from build123d import *

# Parameters (mm, degrees)
F1_DEPTH = 150
F2_R     = 30


with BuildPart() as f1:
    # F0 (on Front) → F1 (new body)
    with BuildSketch(Plane.XZ):
        Polygon((0, 206.360267), (0, 150), (150, 150), (500, 550), (350, 550), (300.684766, 550), align=None)
    extrude(amount=F1_DEPTH)

    # F2
    f2_edges = [f1.edges().sort_by_distance(p)[0] for p in [
        (150.342383, -150, 378.180134),
        (325, -150, 350),
        (325, 0, 350),
        (150.342383, 0, 378.180134),
    ]]
    fillet(f2_edges, radius=F2_R)


solid = f1.part
Design review of the part built by this model. Coordinates are the model's own, in mm. Round coordinates to 2 decimals unless told otherwise and drop trailing zeros. Order: outer loops, then holes, each group sorted by start corner. A loop starts at its lowest first (then second) coordinate and runs counter-clockwise, first axis right, second up.
1) For L1, parallel to X at y = -12, z = 491; L2, parallel to Z at x = 74, y = -74; L3, parallel to X at y = -97.5, z = 197.5, list the stretches that pass through material, from the lowest coordinate up.
The answers:
L1: x = 257.03 to 440.4
L2: z = 150 to 290.93
L3: x = 0 to 191.56
2) Consider section B-B (y = -128). State the section outline as (x, z) points.
The answers:
outline: (0, 150) - (148.56, 150) - (498.56, 550) - (302.13, 550) - (0, 204.71) - close
3) Clearance check with flat-ended pins moving along their axes: pin 1 Ø1 at (y, z) = (-110.5, 274.5) entering from -X; pin 2 Ø1.5 at (y, z) = (-101, 489.5) entering from +X; pin 3 Ø1.5 at (y, z) = (-94.5, 412.5) entering from +X. State where each tip first meets the part, or that it passes through.
The answers:
pin 1: stops at x = 59.18
pin 2: stops at x = 447.72
pin 3: stops at x = 380.34
4) Consider section A-A (y = -52). State the section outline as (x, z) points.
The answers:
outline: (0, 150) - (150, 150) - (500, 550) - (300.68, 550) - (0, 206.36) - close
